Work out the finished part from the listing and answer in its coordinate system (mm). Face numbers are marked on the shaded views. A direction names the side the tool comes from. Coordinates: 2 decimals unless noted, no trailing zeros. Order: outer loops, then holes, each group sorted by start corner. A loop starts at its lowest first (then second) coordinate and runs counter-clockwise, first axis right, second up. Notation, with made-up numbers: M 2,82 L 47,82 A19 cw 47,115 Z; hole C 25.5,59.25 d1. An arc over 180 degrees is marked long. Write item = value, one per line. Start each with the question number.
Q1. Find section C-C on x = -2.25. Give the vertices of the cut face in (y, z).
Q2. A tool of negligible diameter and unlimited length cuts with its end or side. For the marked faces 4, 5 and 6, from which of +Z, -Z, +X, -X, +Y, -Y can it reach the whole face along a straight path? Write none if from no direction.
Q3. Find section D-D on y = 12.5. Give the vertices of the cut face in (x, z).
Q4. Find section A-A on x = -7.5. Give the vertices of the cut face in (y, z), and give its area (3 significant figures).
Q5. Determine the mould class of the marked faces 1, 2 and 3 for opening direction Y: released by +Y, released by -Y, zero draft, split by the parting line, or undercut.
Q6. Each of these flat-tipped pins is pushed along its axis until it touches: P1, Ø1.8, axis at x = -12, y = 3, coming from the -Z side; P2, Ø0.8, axis at x = -2, y = 13, coming from the -Z side; P3, Ø5, axis at x = -7.5, y = 8.5, coming from the +Z side. Where does it stop, or does it pass through?
Q7. Straight lines are drawn through the part: line 1 along Y through (x, z) = (-12, 1.1); line 2 along X through (y, z) = (14.75, 4.25); line 3 along Y through (x, z) = (-3.5, 1.5). For each, find the intervals that lie inside material, in ascending order.
Q8. Find section B-B on y = 3. Give the vertices of the cut face in (x, z).
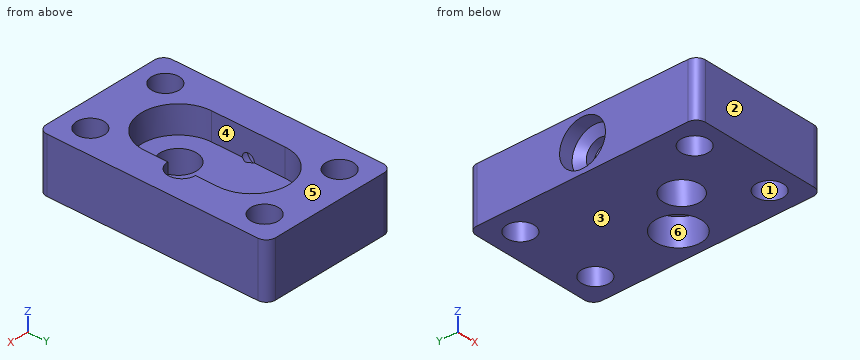
Autodesk Inventor part; units mm, degrees
ref_plane "YZ Plane" through (0, 0, 0) normal (1, 0, 0) x (0, 1, 0)
ref_plane "XZ Plane" through (0, 0, 0) normal (0, 1, 0) x (-1, 0, 0)
ref_plane "XY Plane" through (0, 0, 0) normal (0, 0, 1) x (1, 0, 0)
sketch "Szkic1" plane through (0, 0, 0) normal (0, 0, 1) x (1, 0, 0)
  line L0 (-1, 0) -> (-14, 0)
  line L1 (-15, 1) -> (-15, 24)
  line L2 (-14, 25) -> (-1, 25)
  line L3 (0, 24) -> (0, 1)
  arc A0 (-14, 25) -> (-15, 24) centre (-14, 24) ccw
  arc A1 (0, 24) -> (-1, 25) centre (-1, 24) ccw
  arc A2 (-1, 0) -> (0, 1) centre (-1, 1) ccw
  arc A3 (-15, 1) -> (-14, 0) centre (-14, 1) ccw
  circle A4 centre (-3, 3) radius 1.5
  circle A5 centre (-12, 3) radius 1.5
  circle A6 centre (-12, 22) radius 1.5
  circle A7 centre (-3, 22) radius 1.5
  circle A8 centre (-7.5, 8.5) radius 2
  circle A9 centre (-3.5, 12.5) radius 2.5
  point P0 (0, 0)
  point P1 (-15, 25)
  point P2 (-15, 0)
  point P3 (0, 25)
  point P4 (-11.5, 20.5)
  point P5 (-11.5, 4.5)
  point P6 (-3.5, 20.5)
  dimension "d0" = 15
  dimension "d1" = 25
  dimension "d2" = 1
  dimension "d3" = 3
  dimension "d4" = 3
  dimension "d5" = 3
  dimension "d6" = 3
  dimension "d7" = 8
  dimension "d8" = 16
  dimension "d10" = 19
  dimension "d11" = 4
  dimension "d72" = 5
extrude "Wyciągnięcie proste2" add sketch "Szkic1" along normal blind 3
sketch "Szkic12" plane through (0, 0, 3) normal (0, 0, 1) x (1, 0, 0)
  line L0 (-1, 0) -> (-14, 0)
  line L1 (-15, 1) -> (-15, 24)
  line L2 (-14, 25) -> (-1, 25)
  line L3 (0, 24) -> (0, 1)
  arc A0 (-14, 25) -> (-15, 24) centre (-14, 24) ccw
  arc A1 (0, 24) -> (-1, 25) centre (-1, 24) ccw
  arc A2 (-1, 0) -> (0, 1) centre (-1, 1) ccw
  arc A3 (-15, 1) -> (-14, 0) centre (-14, 1) ccw
  circle A4 centre (-3, 3) radius 1.5
  circle A5 centre (-12, 3) radius 1.5
  circle A6 centre (-12, 22) radius 1.5
  circle A7 centre (-3, 22) radius 1.5
  circle A8 centre (-7.5, 8.5) radius 2
  circle A9 centre (-3.5, 12.5) radius 2.5
  line L4 (-7.5, 4.5) -> (-7.5, 4.5)
  line L5 (-11.5, 8.5) -> (-11.5, 16.5)
  line L6 (-7.5, 20.5) -> (-7.5, 20.5)
  line L7 (-3.5, 16.5) -> (-3.5, 8.5)
  arc A10 (-7.5, 20.5) -> (-11.5, 16.5) centre (-7.5, 16.5) ccw
  arc A11 (-3.5, 16.5) -> (-7.5, 20.5) centre (-7.5, 16.5) ccw
  arc A12 (-7.5, 4.5) -> (-3.5, 8.5) centre (-7.5, 8.5) ccw
  arc A13 (-11.5, 8.5) -> (-7.5, 4.5) centre (-7.5, 8.5) ccw
  arc A14 (-3.5, 11) -> (-3.5, 14) centre (-3.5, 12.5) ccw
  point P0 (0, 0)
  point P1 (0, 0)
  point P2 (-15, 25)
  point P3 (-15, 0)
  point P4 (0, 25)
  point P5 (-11.5, 20.5)
  point P6 (-11.5, 4.5)
  point P7 (-3.5, 20.5)
  point P8 (-11.5, 4.5)
  point P9 (-3.5, 20.5)
  dimension "d38" = 15
  dimension "d39" = 25
  dimension "d40" = 1
  dimension "d41" = 3
  dimension "d42" = 3
  dimension "d43" = 3
  dimension "d44" = 3
  dimension "d45" = 8
  dimension "d46" = 16
  dimension "d47" = 19
  dimension "d48" = 4
  dimension "d49" = 8
  dimension "d50" = 16
  dimension "d51" = 4
  dimension "d52" = 3
extrude "Wyciągnięcie proste3" add sketch "Szkic12" along normal blind 3 contours L0 A3 L1 A0 L2 A1 L3 A2 | A9 L7 A14
sketch "Szkic16" plane through (-15, 1, 0) normal (-1, 0, 0) x (0, 0, 1)
  circle A0 centre (3, 11.5) radius 2.5
  line L0 (0, 14) -> (0, 9)
  point P0 (0, -1)
  dimension "d55" = 5
hole "Otwór2" at (-15, 12.5, 3) direction (1, 0, 0) diameter 5 depth 1.5 tip angle 118
sketch "Szkic17" plane through (-15, 1, 0) normal (-1, 0, 0) x (0, 0, 1)
  line L0 (3, 14) -> (3, 9)
  circle A0 centre (3, 11.5) radius 1.5
  point P0 (0, -1)
  dimension "d64" = 3
hole "Otwór3" at (-15, 12.5, 3) direction (1, 0, 0) diameter 3 depth 3 tip angle 118
properties part number "zad 7"
Findings below:
q1.outline = M 0,0 L 1.7,0 L 1.7,6 L 0,6 Z; M 4.3,0 L 10.33,0 L 10.33,3 L 11.67,3 L 11.67,6 L 4.3,6 Z; M 13.33,3 L 14.67,3 L 14.67,0 L 20.7,0 L 20.7,6 L 13.33,6 Z; M 23.3,0 L 25,0 L 25,6 L 23.3,6 Z
q2.face_4 = +Z
q2.face_5 = +Z, +X, -X, +Y, -Y
q2.face_6 = -Z
q3.outline = M -15,0 L -6,0 L -6,3 L -11.1,3 L -12,1.5 L -12.9,1.5 L -13.5,0.5 L -15,0.5 Z; M -15,5.5 L -13.5,5.5 L -12.9,4.5 L -12,4.5 L -11.5,3.67 L -11.5,6 L -15,6 Z; M -2,3 L -1,3 L -1,0 L 0,0 L 0,6 L -2,6 Z
q4.outline = M 0,0 L 6.5,0 L 6.5,3 L 4.5,3 L 4.5,6 L 0,6 Z; M 10.5,0 L 25,0 L 25,6 L 20.5,6 L 20.5,3 L 10.5,3 Z
q4.area = 90.0 mm^2
q5.face_1 = undercut
q5.face_2 = released by -Y
q5.face_3 = zero draft
q6.P1 = through
q6.P2 = 3
q6.P3 = 3
q7.line_1 = 0 to 1.5, 4.5 to 20.5, 23.5 to 25
q7.line_2 = -15 to -11.5, -3.5 to 0
q7.line_3 = 0 to 1.59, 4.41 to 10, 15 to 20.59, 23.41 to 25
q8.outline = M -15,0 L -13.5,0 L -13.5,6 L -15,6 Z; M -10.5,0 L -4.5,0 L -4.5,6 L -10.5,6 Z; M -1.5,0 L 0,0 L 0,6 L -1.5,6 Z
